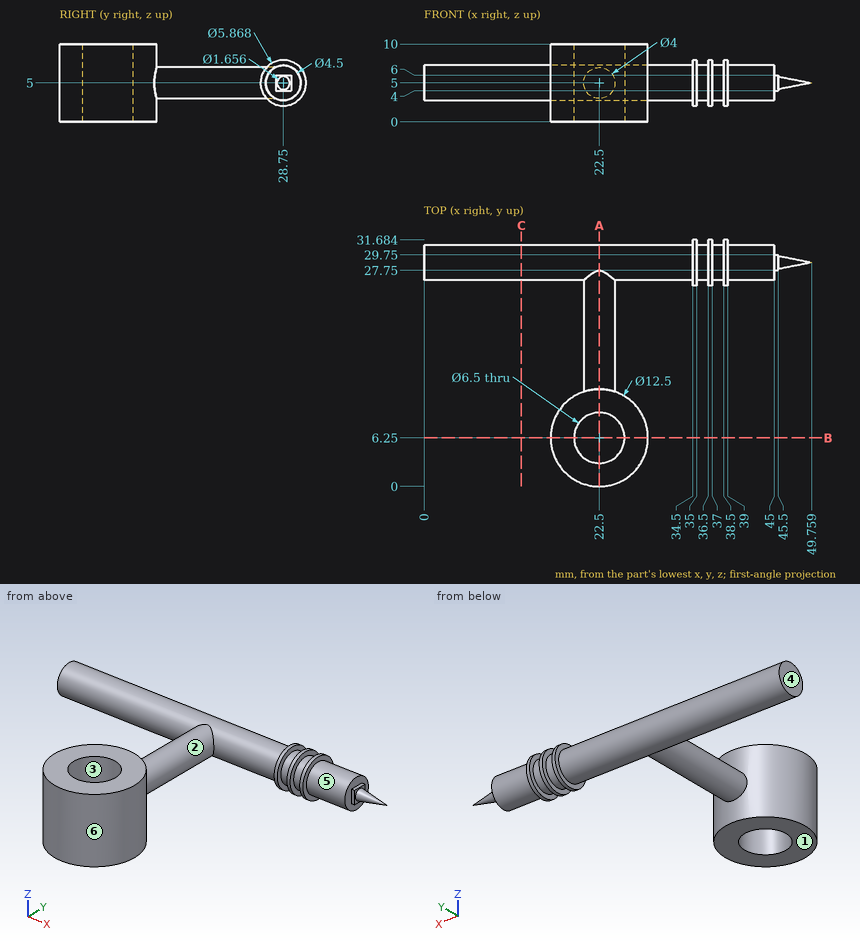
Source: three-view drawing plus pictorial views. Frame: mm from the lowest corner of the part. A direction names the side the tool comes from. Give positions to 0.01 mm unless a question says otherwise; leave off trailing zeros. Write each loop counter-clockwise with the first axis right and the second up, starting at its lowest first coordinate (ties: lowest second). Pieces come first, ordered by that corner, then holes. Notation, with made-up numbers: (-14.75, 77) - (13.25, 77) arc R24 cw to (13.25, 98) - close; hole circle Ø6 at (-18, 2.5). An arc over 180 degrees is marked (long way). Write item = value, one per line. Start each with the question number.
Q1. Cut plane B-B, the plane y = 6.25. Return loops of the section in (x, z).
Q2. Reachability of the marked faces 1 and 2 from +Z, -Z, +X, -X, +Y, -Y: full face, straight path, thin tool, end or side. Return the list, or none.
Q3. Cut plane C-C, the plane x = 12.5. Return loops of the section in (y, z), then the cut area to 3 significant figures.
Q4. Cut plane A-A, the plane x = 22.5. Return loops of the section in (y, z).
Q5. Pin query (flat end, axial travel): pin 1 Ø0.6 at (x, z) = (45, 5) entering from +Y; pin 2 Ø6 at (y, z) = (6.5, 4.5) entering from -X; pin 3 Ø5 at (x, z) = (42, 2) entering from +Y. Return the tip coordinate at first contact, or that it passes through.
Q6. Draft query along Y for the marked faces 3, 4, 5 and 6. Return one class per face: +Y half, -Y half, draft (parallel to the pull), parting line (faces both ways), or undercut.
Q7. Material intervals for probe 1 along Y at (x, z) = (22.5, 8); probe 2 along X at (y, z) = (6.5, 4) (1 decimal); probe 3 along Y at (x, z) = (21.5, 7) (1 decimal), sorted ascending.
Computed values:
q1.outline = (16.25, 0) - (19.25, 0) - (19.25, 10) - (16.25, 10) - close; (25.75, 0) - (28.75, 0) - (28.75, 10) - (25.75, 10) - close
q2.face_1 = -Z, +X, -X, +Y, -Y
q2.face_2 = none
q3.outline = circle Ø4.5 at (28.75, 5)
q3.area = 15.9 mm²
q4.outline = (0, 0) - (3, 0) - (3, 10) - (0, 10) - close; (9.5, 0) - (12.5, 0) - (12.5, 3) - (27.72, 3) arc R2.25 ccw (long way) to (27.72, 7) - (12.5, 7) - (12.5, 10) - (9.5, 10) - close
q5.pin_1 = 31
q5.pin_2 = 16.25
q5.pin_3 = 30.94
q6.face_3 = undercut
q6.face_4 = draft
q6.face_5 = parting line
q6.face_6 = undercut
q7.probe_1 = 0 to 3, 9.5 to 12.5
q7.probe_2 = 16.3 to 19.3, 25.7 to 28.7
q7.probe_3 = 0.1 to 3.2, 9.3 to 12.4, 27.7 to 29.8
